For this review, take the finished solid that the model builds, in its own axes (mm). Face numbers are marked on the shaded views. A direction names the side the tool comes from. Give positions to 0.01 mm unless a question says otherwise; leave off trailing zeros. Order: outer loops, then holes, each group sorted by start corner. A loop starts at its lowest first (then second) coordinate and runs counter-clockwise, first axis right, second up. Notation, with made-up numbers: (-34, 8.25) -> (12, 8.25) arc R23 cw to (12, 21.25) -> close; hole circle Ø5 at (19.5, 77.25). An arc over 180 degrees is marked (long way). Return JSON: item names as keys, results as strings. Group by question number.
1) Add section D-D (y = 28.5). Give the boundary of the cut face in (x, z).
2) To check wall thickness, follow line 1 along Z through (x, y) = (27.5, 5.5); line 2 along Y through (x, z) = (55.5, -7); line 3 along Z through (x, y) = (47, 15). State the ranges of each line that lie inside material, in increasing order.
3) Add section C-C (x = 59.5). Give the boundary of the cut face in (y, z).
4) Add section A-A (y = 4). Give the boundary of the cut face in (x, z), then the cut area to 3 significant figures.
5) Add section B-B (z = 19.5). Give the boundary of the cut face in (x, y).
6) For the marked faces 1, 2 and 3, list the 3-axis set-ups (+Z, -Z, +X, -X, +Y, -Y) from which the entire face can be reached by the end or side of a thin tool; tool diameter is ignored.
7) Insertion check: P1, Ø1, axis at x = 16.5, z = -4.5, coming from the +Y side; P2, Ø6, axis at y = 33, z = 7.5, coming from the -X side; P3, Ø5, axis at x = 12, y = 5, coming from the +Z side. Each pin has a flat end and moves straight along its axis. Give the tip position at first contact, or say it passes through.
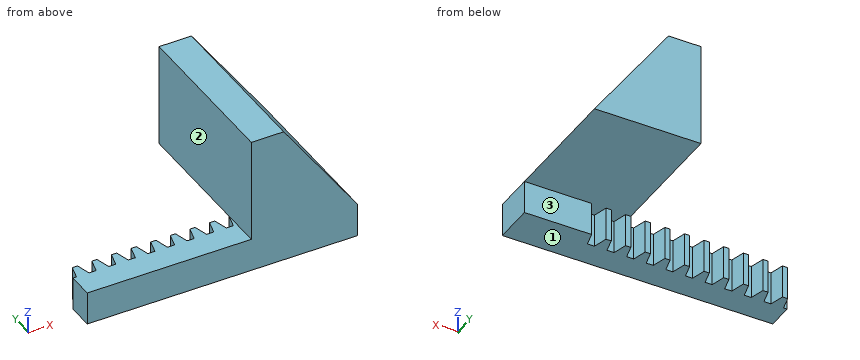
from build123d import *

# Parameters (mm, degrees)
BLANKSKE_W          = 50
BLANKSKE_H          = 9.5
BLANK_DEPTH         = 8
TOOTHCUTSIM_DEPTH   = 52.519413817
TEETHCUTS_COUNT     = 11
TEETHCUTS_PITCH     = 4.712388975
SKETCH3_W           = 8
SKETCH3_H           = 9.5
BOSS_EXTRUDE2_DEPTH = 15
BOSS_EXTRUDE5_DEPTH = 39.5


with BuildPart() as part:
    # BlankSke → Blank (new body)
    with BuildSketch(Plane.XY):
        with Locations((25, 4.75)):
            Rectangle(BLANKSKE_W, BLANKSKE_H)
    extrude(amount=-BLANK_DEPTH)

    # TooCutSkeSim → ToothCutSim (cut, through all)
    with BuildSketch(Plane.XY):
        Polygon((0.852189273, 6.125), (-0.852189273, 6.125), (-1.731592507, 9.5254), (1.731592507, 9.5254), align=None)
    toothcutsim = extrude(amount=-TOOTHCUTSIM_DEPTH, mode=Mode.SUBTRACT)

    # TeethCuts: ToothCutSim ×11
    with Locations(*[(i * TEETHCUTS_PITCH, 0, 0) for i in range(1, TEETHCUTS_COUNT)]):
        add(toothcutsim, mode=Mode.SUBTRACT)

    # Sketch3 → Boss-Extrude2 (add)
    with BuildSketch(Plane(origin=(50, 0, 0), x_dir=(0, 0, -1), z_dir=(1, 0, 0))):
        with Locations((4, 4.75)):
            Rectangle(SKETCH3_W, SKETCH3_H)
    extrude(amount=BOSS_EXTRUDE2_DEPTH)

    # Sketch7 → Boss-Extrude5 (add)
    with BuildSketch(Plane(origin=(0, 0, 0), x_dir=(1, 0, 0), z_dir=(0, 1, 0))):
        Polygon((65, 0), (39.42413542, 0), (39.42413542, -25), (47.21206771, -25), align=None)
    extrude(amount=BOSS_EXTRUDE5_DEPTH)


solid = part.part
Evaluation:
{
 "1": {"outline": "(39.42, 0) -> (65, 0) -> (47.21, 25) -> (39.42, 25) -> close"},
 "2": {"line 1": "-8 to 0", "line 2": "0 to 9.5", "line 3": "0 to 25"},
 "3": {"outline": "(0, -8) -> (9.5, -8) -> (9.5, 0) -> (39.5, 0) -> (39.5, 7.73) -> (0, 7.73) -> close"},
 "4": {"outline": "(0, -8) -> (65, -8) -> (65, 0) -> (47.21, 25) -> (39.42, 25) -> (39.42, 0) -> (0, 0) -> close", "area": "937 mm^2"},
 "5": {"outline": "(39.42, 0) -> (51.13, 0) -> (51.13, 39.5) -> (39.42, 39.5) -> close"},
 "6": {"face 1": "-Z, +X, -X, +Y, -Y", "face 2": "+Z, -X, +Y, -Y", "face 3": "-Z, +X, -X, +Y"},
 "7": {"P1": "y = 9.5", "P2": "x = 39.42", "P3": "z = 0"}
}
